Build history of the part. All positions in model axes, mm. A direction names the side the tool comes from. Coordinates: 2 decimals unless noted, no trailing zeros. Order: outer loops, then holes, each group sorted by start corner. A loop starts at its lowest first (then second) coordinate and runs counter-clockwise, first axis right, second up. Notation, with made-up numbers: (5.5, 2.25) - (36.5, 2.25) arc R19 cw to (36.5, 12.25) - close; hole circle Ø5 at (7.25, 17.25). An arc over 180 degrees is marked (long way). One line per item, written item: value.
Solid Edge part; units mm, degrees
sketch "Sketch1" plane through (0, 0, 0) normal (0, 0, 1) x (1, 0, 0)
  line L0 (-8, -3.5) -> (10, -3.5)
  line L1 (10, -3.5) -> (10, 3.5)
  line L2 (10, 3.5) -> (-8, 3.5)
  line L3 (-8, 3.5) -> (-8, -3.5)
  dimension "D1" = 8
  dimension "D2" = 10
extrude "Protrusion1" add sketch "Sketch1" along normal blind 0.5
sketch "Sketch2" plane through (2, 0, 0.5) normal (0, 0, 1) x (-1, 0, 0)
  line L0 (8.8487, -0.65) -> (3.6487, -0.65)
  line L1 (3.6487, -0.65) -> (3.6487, -1.2914)
  line L2 (3.6487, -1.2914) -> (4.2073, -1.85)
  line L3 (4.2073, -1.85) -> (8.2901, -1.85)
  line L4 (8.2901, -1.85) -> (8.8487, -1.2914)
  line L5 (8.8487, -1.2914) -> (8.8487, -0.65)
extrude "Cutout1" cut sketch "Sketch2" against normal up to next
sketch "Sketch3" plane through (2, 0, 0) normal (0, 0, -1) x (1, 0, 0)
  line L0 (-8.2901, -1.85) -> (-8.8487, -1.2914)
  line L1 (-8.8487, -1.2914) -> (-8.8487, -0.65)
  line L2 (-8.8487, -0.65) -> (-3.6487, -0.65)
  line L3 (-3.6487, -0.65) -> (-3.6487, -1.2914)
  line L4 (-3.6487, -1.2914) -> (-4.2073, -1.85)
  line L5 (-4.2073, -1.85) -> (-8.2901, -1.85)
  line L6 (-9.1987, -0.3) -> (-3.2987, -0.3)
  line L7 (-3.2987, -0.3) -> (-3.2987, -1.4364)
  line L8 (-3.2987, -1.4364) -> (-4.0623, -2.2)
  line L9 (-4.0623, -2.2) -> (-8.4351, -2.2)
  line L10 (-8.4351, -2.2) -> (-9.1987, -1.4364)
  line L11 (-9.1987, -1.4364) -> (-9.1987, -0.3)
extrude "ExtrudedProtrusion_2" add sketch "Sketch3" along normal blind 1.25
sketch "Sketch4" plane through (-3.0487, 2.2, -0.625) normal (0, 1, 0) x (1, 0, 0)
  line L0 (-0.05, -0.625) -> (-0.05, 1.2393)
  line L1 (-0.3, 1.2393) -> (-0.05, 1.2393)
  line L2 (-0.3, -0.625) -> (-0.3, 1.2393)
  line L3 (-0.05, -0.625) -> (-0.3, -0.625)
  line L4 (-2.55, 1.2393) -> (-2.55, -0.625)
  line L5 (-2.3, -0.625) -> (-2.55, -0.625)
  line L6 (-2.3, 1.2393) -> (-2.3, -0.625)
  line L7 (-2.55, 1.2393) -> (-2.3, 1.2393)
extrude "Cutout2" cut sketch "Sketch4" against normal up to next
sketch "Sketch5" plane through (-3.3487, 2.025, -0.625) normal (1, 0, 0) x (0, -1, 0)
  line L0 (0.175, -0.1) -> (0.425, -0.1)
  line L1 (0.425, -0.1) -> (0.175, 0.625)
  dimension "D1" = 0.175
extrude "Protrusion2" add sketch "Sketch5" against normal up to vertex (2 mm away) material side at (-3.3487, 1.725, -0.575)
fillet "Round_1" radius 0.05 1 edges at (-4.3487, 1.6, -0.525)
fillet "Round_2" radius 1 4 edges at (10, 3.5, 0.25) (10, -3.5, 0.25) (-8, 3.5, 0.25) (-8, -3.5, 0.25)
sketch "Sketch6" plane through (2, 0, 0.5) normal (0, 0, 1) x (-1, 0, 0)
  circle A0 centre (-3, -1) radius 0.5
  circle A1 centre (-3, 1) radius 0.5
  dimension "D1" = 3
extrude "ExtrudedProtrusion_4" add sketch "Sketch6" along normal blind 0.5
sketch "Sketch7" plane through (2, 0, 0.5) normal (0, 0, 1) x (-1, 0, 0)
  line L0 (-3.875, -2) -> (-2.125, -2)
  line L1 (-2.125, -2) -> (-2.125, 2)
  line L2 (-2.125, 2) -> (-3.875, 2)
  line L3 (-3.875, 2) -> (-3.875, -2)
  dimension "D1" = 2.125
  dimension "D2" = 3.875
extrude "ExtrudedProtrusion_5" add sketch "Sketch7" along normal blind 0.15
fillet "Round_3" radius 0.25 4 edges at (5.875, 2, 0.575) (4.125, 2, 0.575) (4.125, -2, 0.575) (5.875, -2, 0.575)
sketch "Sketch8" plane through (6, 1.5, 0.575) normal (0, 1, 0) x (-1, 0, 0)
  line L0 (1.875, 0.075) -> (8.6082, 1.9893)
  line L1 (8.6082, 1.9893) -> (9.1082, 1.9893)
  line L2 (9.1082, 1.9893) -> (9.1082, 1.8505)
  line L3 (9.1082, 1.8505) -> (8.6476, 1.8505)
  line L4 (1.875, -0.075) -> (8.6476, 1.8505)
  dimension "D1" = 1.875
  dimension "D2" = 8.6082
extrude "ExtrudedProtrusion_6" add sketch "Sketch8" against normal blind 0.75 material side at (0.7447, 1.5, 1.5591)
fillet "Round_4" radius 0.25 2 edges at (-3.1082, 1.5, 2.4949) (-3.1082, 0.75, 2.4949)
mirror "Mirror1" about plane through (6, 0, 0.575) normal (0, 1, 0) of "ExtrudedProtrusion_6"
fillet "Round1" radius 0.25 2 edges at (-3.1082, -1.5, 2.4949) (-3.1082, -0.75, 2.4949)
mirror "Mirror2" about plane through (5, 0, 0.575) normal (1, 0, 0) of "Mirror1", "ExtrudedProtrusion_6"
fillet "Round2" radius 0.25 2 edges at (13.1082, 1.5, 2.4949) (13.1082, 0.75, 2.4949)
fillet "Round3" radius 0.25 2 edges at (13.1082, -1.5, 2.4949) (13.1082, -0.75, 2.4949)
properties material "Polypropylene, general purpose"
1. Two-plate mould, pull along Y, no slides. Class faces 1 (the face through (-4, 1.85, 0)), 2 (the face through (-6, 2.2, -1)), 3 (the face through (5, -1, 1)): pulls with the +Y half, pulls with the -Y half, needs draft (parallel to the pull), parting line crosses it, or undercut.
Values found:
face 1: undercut
face 2: pulls with the +Y half
face 3: needs draft
2. Band-saw the part on C-C, the plane y = -0.25. Give the cut face in (x, z) (3 decimals).
Values found:
outline: (-8, 0) - (10, 0) - (10, 0.5) - (5.875, 0.5) - (5.875, 0.65) - (4.125, 0.65) - (4.125, 0.5) - (-8, 0.5) - close
3. Band-saw the part on D-D, the plane z = 1.8. Give the cut face in (x, y).
Values found:
outline: (-0.45, -1.5) - (0.08, -1.5) - (0.08, -0.75) - (-0.45, -0.75) - close; (-0.45, 0.75) - (0.08, 0.75) - (0.08, 1.5) - (-0.45, 1.5) - close; (9.92, -1.5) - (10.45, -1.5) - (10.45, -0.75) - (9.92, -0.75) - close; (9.92, 0.75) - (10.45, 0.75) - (10.45, 1.5) - (9.92, 1.5) - close
4. Flat gauge pins, fed straight in: P1, Ø1, axis at x = 4, y = -0.5, coming from the +Z side; P2, Ø0.6, axis at x = 2, z = 1, coming from the -Y side; P3, Ø0.5, axis at x = -3, y = -1, coming from the -Z side; P4, Ø1.5, axis at x = -4.5, z = 1, coming from the +Y side. Where does each tip first touch, or does it go through?
Values found:
P1: stops at z = 0.81
P2: stops at y = -1.5
P3: stops at z = 0
P4: stops at y = 3.5
5. Band-saw the part on B-B, the plane x = 1.75. Give the cut face in (y, z).
Values found:
outline: (-3.5, 0) - (3.5, 0) - (3.5, 0.5) - (-3.5, 0.5) - close; (-1.5, 1.18) - (-0.75, 1.18) - (-0.75, 1.33) - (-1.5, 1.33) - close; (0.75, 1.18) - (1.5, 1.18) - (1.5, 1.33) - (0.75, 1.33) - close
6. 3-axis set-ups, long thin cutter, end or side, ignore diameter. For faces 4 (the face through (5.4, 0.7, 0.8)), 5 (the face through (9.715, 3.199, 0.254)): which of +Z, -Z, +X, -X, +Y, -Y reach the whole face in a straight line?
Values found:
face 4: +Z
face 5: +Z, -Z, +X, +Y
7. Band-saw the part on A-A, the plane x = 10.5. Give the cut face in (y, z), and give its area (3 significant figures).
Values found:
outline: (-1.5, 1.81) - (-0.75, 1.81) - (-0.75, 1.96) - (-1.5, 1.96) - close; (0.75, 1.81) - (1.5, 1.81) - (1.5, 1.96) - (0.75, 1.96) - close
area: 0.225 mm2
8. Probe line 1 along Y through (x, z) = (-5.5, 0.05); line 2 along Z through (x, y) = (-6, -1.25); line 3 along Z through (x, y) = (9.25, 1.25). List the from-to ranges inside material, lowest first.
Values found:
line 1: y = -3.5 to 0.65, 1.85 to 3.5
line 2: z = 0 to 0.5
line 3: z = 0 to 0.5, 1.46 to 1.61
